```python
from build123d import *

# Parameters (mm, degrees)
F0_W     = 12
F0_H     = 12
F0_R     = 1.7
F1_DEPTH = 12
F2_R     = 1.7
F3_DEPTH = 12
F4_R     = 1.7
F5_DEPTH = 12


with BuildPart() as f1:
    # F0 (on Top) → F1 (new body)
    with BuildSketch(Plane.XY):
        Rectangle(F0_W, F0_H)
        Circle(F0_R, mode=Mode.SUBTRACT)
    extrude(amount=F1_DEPTH)

    # F2 (on face) → F3 (cut)
    with BuildSketch(Plane(origin=(-6, 0, 0), x_dir=(0, -1, 0), z_dir=(-1, 0, 0))):
        with Locations((0, 6)):
            Circle(F2_R)
    extrude(amount=-F3_DEPTH, mode=Mode.SUBTRACT)

    # F4 (on face) → F5 (cut)
    with BuildSketch(Plane(origin=(0, 6, 0), x_dir=(-1, 0, 0), z_dir=(0, 1, 0))):
        with Locations((0, 6)):
            Circle(F4_R)
    extrude(amount=-F5_DEPTH, mode=Mode.SUBTRACT)


solid = f1.part
```
Input: part model. Units: mm. Frame: model coordinates. Coordinates: 2 decimals unless noted, no trailing zeros. Loops run counter-clockwise (first coordinate to the right, second up) from the corner with the lowest first, then second, coordinate; pieces in that order, holes last.
Q1. Contact query for a flat-ended pin moving along its axis: pin 1 (6 mm diameter, centred on x = 1.5, y = -4, fed in from -Z). Output: stop coordinate, or through.
Results are:
pin 1: stops at z = 0
Q2. Mould query, pull axis Z, two halves, no side actions, for faces 1 (the cylindrical face through (-1.25, 1.15, 2.37)), 2 (the cylindrical face through (1.25, -3.57, 7.15)), 3 (the flat face through (1.25, 1.42, 12)), 4 (the flat face through (1.25, 1.42, 0)). Classes: +Z half, -Z half, draft (parallel to the pull), parting line (faces both ways), or undercut.
Results are:
face 1: draft
face 2: undercut
face 3: +Z half
face 4: -Z half
Q3. Section A-A, the plane x = 0. Return the cut outline in (y, z), and give its area (3 significant figures).
Results are:
outline: (-6, 0) - (-1.7, 0) - (-1.7, 4.3) - (-6, 4.3) - close; (-6, 7.7) - (-1.7, 7.7) - (-1.7, 12) - (-6, 12) - close; (1.7, 0) - (6, 0) - (6, 4.3) - (1.7, 4.3) - close; (1.7, 7.7) - (6, 7.7) - (6, 12) - (1.7, 12) - close
area: 74.0 mm2
Q4. Section D-D, the plane x = 5. Return the cut outline in (y, z), and give its area (3 significant figures).
Results are:
outline: (-6, 0) - (6, 0) - (6, 12) - (-6, 12) - close; hole circle Ø3.4 at (0, 6)
area: 135 mm2
Q5. Section C-C, the plane z = 1.25. Return the cut outline in (x, y), and give its area (3 significant figures).
Results are:
outline: (-6, -6) - (6, -6) - (6, 6) - (-6, 6) - close; hole circle Ø3.4 at (0, 0)
area: 135 mm2
Q6. Line query: line 1 along X through (y, z) = (3.7, 6); line 2 along Z through (x, y) = (0, -4.35). Output: solid intervals per line, ascending.
Results are:
line 1: x = -6 to -1.7, 1.7 to 6
line 2: z = 0 to 4.3, 7.7 to 12
